```python
from build123d import *

# Parameters (mm, degrees)
F1_DEPTH      = 11.3
F2_R          = 4.8
F3_DEPTH      = 5.8
F4_R          = 4.125
F5_DEPTH      = 12.45
F6_R          = 3.15
F7_DEPTH      = 23.88
F8_R          = 1
F9_DEPTH      = 6.731
F9_DEPTH_BACK = 6.731
F10_R         = 5.635
F11_DEPTH     = 3.7
F12_R         = 7.25
F12_R_2       = 5.635
F13_DEPTH     = 3.8
F14_R         = 4.75
F15_DEPTH     = 10
F16_W         = 3.3575966954
F16_H         = 14.4844972529
F17_DEPTH     = 16
F18_R         = 1.295
F19_DEPTH     = 4.37


with BuildPart() as f1:
    # F0 (on Front) → F1 (new body)
    with BuildSketch(Plane.XZ):
        with BuildLine():
            ThreePointArc((6.73, 11.5308485135), (0, 18.2608485135), (-6.73, 11.5308485135))
            Line((-6.73, 11.5308485135), (-6.73, -4.5823248016))
            Line((-6.73, -4.5823248016), (6.73, -4.5823248016))
            Line((6.73, -4.5823248016), (6.73, 11.5308485135))
        make_face()
    extrude(amount=-F1_DEPTH)

    # F2 (on face) → F3 (join)
    with BuildSketch(Plane.XZ):
        with Locations((0, 11.5308485135)):
            Circle(F2_R)
    extrude(amount=F3_DEPTH)

    # F4 (on face) → F5 (join)
    with BuildSketch(Plane.XZ):
        with Locations((0, 11.5308485135)):
            Circle(F4_R)
    extrude(amount=F5_DEPTH)

    # F6 (on face) → F7 (join)
    with BuildSketch(Plane.XZ):
        with Locations((0, 11.5308485135)):
            Circle(F6_R)
    extrude(amount=F7_DEPTH)

    # F8 (on Right) → F9 (cut, two sides)
    with BuildSketch(Plane.YZ) as f9_sk:
        with Locations((-21.5193368495, 11.6681437939)):
            Circle(F8_R)
    extrude(amount=-F9_DEPTH, mode=Mode.SUBTRACT)
    extrude(f9_sk.sketch, amount=F9_DEPTH_BACK, mode=Mode.SUBTRACT)

    # F10 (on face) → F11 (join)
    with BuildSketch(Plane(origin=(0, 11.3, 0), x_dir=(-1, 0, 0), z_dir=(0, 1, 0))):
        with Locations((0, 11.5308485135)):
            Circle(F10_R)
    extrude(amount=F11_DEPTH)

    # F12 (on face) → F13 (join)
    with BuildSketch(Plane(origin=(0, 15, 0), x_dir=(-1, 0, 0), z_dir=(0, 1, 0))):
        with Locations((0, 11.5308485135)):
            Circle(F12_R)
        with Locations((0, 11.5308485135)):
            Circle(F12_R_2, mode=Mode.SUBTRACT)
        with Locations((0, 11.5308485135)):
            Circle(F12_R_2)
    extrude(amount=F13_DEPTH)

    # F14 (on face) → F15 (join)
    with BuildSketch(Plane.YZ.offset(6.73)):
        with Locations((5.65, 1.4176751984)):
            Circle(F14_R)
    extrude(amount=F15_DEPTH)

    # F16 (on face) → F17 (join)
    with BuildSketch(Plane.YZ.offset(16.73)):
        with Locations((5.616213195, 0.8844293188)):
            Rectangle(F16_W, F16_H)
    extrude(amount=F17_DEPTH)

    # F18 (on face) → F19 (join)
    with BuildSketch(Plane.XZ):
        with Locations((0, -1.5323248016)):
            Circle(F18_R)
    extrude(amount=F19_DEPTH)


solid = f1.part
```
Can you work these out from the model? Positions are in its coordinate system, mm. A direction names the side the tool comes from. Round coordinates to 2 decimals unless told otherwise and drop trailing zeros. Loops run counter-clockwise (first coordinate to the right, second up) from the corner with the lowest first, then second, coordinate; pieces in that order, holes last. Notation, with made-up numbers: (77.25, 75.25) -> (103.25, 75.25) arc R15 cw to (103.25, 81.25) -> close; hole circle Ø6 at (13.25, -6.75). An arc over 180 degrees is marked (long way). Answer in a Markdown table with one row per item.
Item 1: We'd pull the mould along X, two halves only. Please class faces 6 (the flat face through (16.73, 6, -5)), 7 (the cylindrical face through (-0.894, -9.078, 7.504)), 8 (the flat face through (0, 18.8, 12)): released by +X, released by -X, zero draft, split by the parting line, or undercut.
Answer block:
| item | result |
|---|---|
| face 6 | undercut |
| face 7 | split by the parting line |
| face 8 | zero draft |
Item 2: If I drill on probe 1 along Y at (x, z) = (-2, 16.5); probe 2 along X at (y, z) = (3, 0.75); probe 3 along Y at (x, z) = (23.5, 1.5), over which ranges is the centre line in solid material (lowest first)?
Answer block:
| item | result |
|---|---|
| probe 1 | 0 to 18.8 |
| probe 2 | -6.73 to 16.73 |
| probe 3 | 3.94 to 7.3 |
Item 3: Will these pins go through, and if not, where does the flat tip stop? P1, Ø1.8, axis at y = -21.52, z = 11.67, coming from the +X side; P2, Ø10, axis at x = 5.5, z = 0, coming from the -Y side; P3, Ø12.5, axis at x = -0.5, y = 6.5, coming from the -Z side; P4, Ø1.1, axis at y = 6.5, z = 7, coming from the -X side.
Answer block:
| item | result |
|---|---|
| P1 | through |
| P2 | y = -4.37 |
| P3 | z = -4.58 |
| P4 | x = -6.73 |
Item 4: Suppose I cut it at A-A, the plane y = 5.65. List the corners of the cut face in (x, z) for me.
Answer block:
| item | result |
|---|---|
| outline | (-6.73, -4.58) -> (6.73, -4.58) -> (6.73, -3.33) -> (16.73, -3.33) -> (16.73, -6.36) -> (32.73, -6.36) -> (32.73, 8.13) -> (16.73, 8.13) -> (16.73, 6.17) -> (6.73, 6.17) -> (6.73, 11.53) arc R6.73 ccw to (-6.73, 11.53) -> close |
Item 5: Suppose I cut it at D-D, the plane y = 13. List the corners of the cut face in (x, z) for me (3 decimals).
Answer block:
| item | result |
|---|---|
| outline | circle Ø11.27 at (0, 11.531) |
Item 6: On a 3-axis mill with a long thin cutter (end or side, diameter ignored), from which of +Z, -Z, +X, -X, +Y, -Y can I reach the whole of each face in a straight line? I mean faces 1 (the flat face through (25, 3.937, 1)), 2 (the flat face through (-6.73, 6, 4)), 3 (the cylindrical face through (-5.375, 13.124, 13.223)), 4 (the flat face through (16.73, 8, 1)), 5 (the cylindrical face through (-0.62, -2.86, 16.29)). Say none if no direction works.
Answer block:
| item | result |
|---|---|
| face 1 | +Z, -Z, +X, -Y |
| face 2 | +Z, -Z, -X, -Y |
| face 3 | none |
| face 4 | +Z, -Z, +X, +Y |
| face 5 | -Y |
Item 7: Suppose I cut it at C-C, the plane z = 2.25. List the corners of the cut face in (x, y) for me, plus the area to 3 significant figures.
Answer block:
| item | result |
|---|---|
| outline | (-6.73, 0) -> (6.73, 0) -> (6.73, 0.97) -> (16.73, 0.97) -> (16.73, 3.94) -> (32.73, 3.94) -> (32.73, 7.3) -> (16.73, 7.3) -> (16.73, 10.33) -> (6.73, 10.33) -> (6.73, 11.3) -> (-6.73, 11.3) -> close |
| area | 299 mm² |
Item 8: Suppose I cut it at B-B, the plane x = 20. List the corners of the cut face in (y, z) for me.
Answer block:
| item | result |
|---|---|
| outline | (3.94, -6.36) -> (7.3, -6.36) -> (7.3, 8.13) -> (3.94, 8.13) -> close |
